```python
from build123d import *

# Parameters (mm, degrees)
SKETCH1_R           = 19.05
SKETCH1_R_2         = 9.525
SKETCH1_R_3         = 1.7526
BOSS_EXTRUDE1_DEPTH = 16.0528
SKETCH2_R           = 11.1125
CUT_EXTRUDE2_DEPTH  = 5.588


with BuildPart() as part:
    # Sketch1 → Boss-Extrude1 (new body)
    with BuildSketch(Plane.XY):
        Circle(SKETCH1_R)
        Circle(SKETCH1_R_2, mode=Mode.SUBTRACT)
        with Locations((0, 15.24)):
            Circle(SKETCH1_R_3, mode=Mode.SUBTRACT)
        with Locations((15.24, 0)):
            Circle(SKETCH1_R_3, mode=Mode.SUBTRACT)
        with Locations((0, -15.24)):
            Circle(SKETCH1_R_3, mode=Mode.SUBTRACT)
        with Locations((-15.24, 0)):
            Circle(SKETCH1_R_3, mode=Mode.SUBTRACT)
    extrude(amount=BOSS_EXTRUDE1_DEPTH)

    # Sketch2 → Cut-Extrude2 (cut)
    with BuildSketch(Plane.XY.offset(16.0528)):
        Circle(SKETCH2_R)
    extrude(amount=-CUT_EXTRUDE2_DEPTH, mode=Mode.SUBTRACT)


solid = part.part
```
Check sheet for the modelled part. Datum: model origin and axes. Units: mm. A direction names the side the tool comes from. Coordinates: 2 decimals unless noted, no trailing zeros. Loops run counter-clockwise (first coordinate to the right, second up) from the corner with the lowest first, then second, coordinate; pieces in that order, holes last.
1) Gauge pin test, flat ends, axial feed: pin 1 (6.5 mm diameter, centred on x = 1, y = 4, fed in from +Z); pin 2 (4 mm diameter, centred on x = 0, y = 15.24, fed in from +Z); pin 3 (3 mm diameter, centred on x = -0.5, z = 2, fed in from -Y); pin 4 (1 mm diameter, centred on y = 3, z = 3.5, fed in from +X). Record the tip position at first contact, or that the pin passes through.
2) Access from +Z, -Z, +X, -X, +Y, -Y to the whole of each face (thin tool, end or side, straight path). Record for faces 1 (the face through (-0.2, -13.5, 7.9)), 2 (the face through (-5, 8.3, 10.465)).
3) Sectioned sample at D-D (x = -5). Record the boundary of the cut face in (y, z).
4) Release check for a two-part mould opening along X. For faces 3 (the face through (10.6, 3.34, 13.3)), 4 (the face through (8, -8, 16.053)), 5 (the face through (-15.12, -11.59, 7.91)) record: released by +X, released by -X, zero draft, split by the parting line, or undercut.
5) Material ranges on probe 1 along X at (y, z) = (1.5, 12.5); probe 2 along Y at (x, z) = (-16, 13.5); probe 3 along Y at (x, z) = (3.5, 5), recorded low to high.
6) Sectioned sample at A-A (y = -15.24). Record the boundary of the cut face in (x, z).
7) Sectioned sample at C-C (z = 7.5). Record the boundary of the cut face in (x, y) (3 decimals), and give its area (3 significant figures).
Check sheet entries:
1. pin 1: passes through
1. pin 2: stops at z = 16.05
1. pin 3: stops at y = -19.05
1. pin 4: stops at x = 18.89
2. face 1: +Z, -Z
2. face 2: +Z
3. outline: (-18.38, 0) - (-8.11, 0) - (-8.11, 10.46) - (-9.92, 10.46) - (-9.92, 16.05) - (-18.38, 16.05) - close; (8.11, 0) - (18.38, 0) - (18.38, 16.05) - (9.92, 16.05) - (9.92, 10.46) - (8.11, 10.46) - close
4. face 3: undercut
4. face 4: zero draft
4. face 5: split by the parting line
5. probe 1: x = -18.99 to -16.15, -14.33 to -11.01, 11.01 to 14.33, 16.15 to 18.99
5. probe 2: y = -10.34 to -1.58, 1.58 to 10.34
5. probe 3: y = -18.73 to -8.86, 8.86 to 18.73
6. outline: (-11.43, 0) - (-1.75, 0) - (-1.75, 16.05) - (-11.43, 16.05) - close; (1.75, 0) - (11.43, 0) - (11.43, 16.05) - (1.75, 16.05) - close
7. outline: circle Ø38.1 at (0, 0); hole circle Ø3.505 at (-15.24, 0); hole circle Ø19.05 at (0, 0); hole circle Ø3.505 at (0, -15.24); hole circle Ø3.505 at (0, 15.24); hole circle Ø3.505 at (15.24, 0)
7. area: 816 mm2
